Autodesk Inventor part; units mm, degrees
ref_plane "YZ Plane" through (0, 0, 0) normal (1, 0, 0) x (0, 1, 0)
ref_plane "XZ Plane" through (0, 0, 0) normal (0, 1, 0) x (-1, 0, 0)
ref_plane "XY Plane" through (0, 0, 0) normal (0, 0, 1) x (1, 0, 0)
sketch "Sketch1" plane through (0, 0, 0) normal (0, 0, 1) x (1, 0, 0)
  line L0 (0, 0) -> (80, 0)
  line L1 (80, 0) -> (80, 50)
  line L2 (80, 50) -> (0, 50)
  line L3 (0, 50) -> (0, 0)
  line L4 (15, 50) -> (65, 50)
  line L5 (65, 50) -> (65, 45)
  line L6 (65, 45) -> (15, 45)
  line L7 (15, 45) -> (15, 50)
  line L8 (5, 40) -> (75, 40)
  line L9 (75, 40) -> (75, 5)
  line L10 (75, 5) -> (5, 5)
  line L11 (5, 5) -> (5, 40)
  line L12 (-10, 0) -> (90, 0)
  line L13 (90, 0) -> (90, 5)
  line L14 (90, 5) -> (-10, 5)
  line L15 (-10, 5) -> (-10, 0)
  line L16 (0, 50) -> (5, 50)
  line L17 (5, 50) -> (5, 45)
  line L18 (5, 45) -> (0, 45)
  line L19 (0, 45) -> (0, 50)
  line L20 (80, 50) -> (75, 50)
  line L21 (75, 50) -> (75, 45)
  line L22 (75, 45) -> (80, 45)
  line L23 (80, 45) -> (80, 50)
  line L24 (37.5, 40) -> (42.5, 40)
  line L25 (42.5, 40) -> (42.5, 5)
  line L26 (42.5, 5) -> (37.5, 5)
  line L27 (37.5, 5) -> (37.5, 40)
  point P0 (40, 50)
  point P1 (40, 5)
  point P2 (40, 0)
  point P3 (40, 40)
  dimension "d0" = 80
  dimension "d1" = 50
  dimension "d2" = 50
  dimension "d3" = 70
  dimension "d4" = 100
  dimension "d5" = 5
  dimension "d6" = 5
  dimension "d7" = 5
  dimension "d10" = 5
  dimension "d11" = 5
  dimension "d12" = 5
extrude "Extrusion1" add sketch "Sketch1" along normal blind 10 contours L3 L14 L10 L1 L0 | L12 L15 L14 L3 | L1 L14 L13 L12 | L3 L18 L17 L2 L7 L6 L5 L21 L22 L1 L14 L9 L8 L11 | L27 L8 L25 L10
sketch "Sketch2" plane through (5, 50, 0) normal (0, 1, 0) x (1, 0, 0)
  line L0 (10, 0) -> (0, 0)
  circle A0 centre (5, -5) radius 1.7
  circle A1 centre (-10, -5) radius 1.7
  circle A2 centre (65, -5) radius 1.7
  circle A3 centre (80, -5) radius 1.7
  line L1 (70, -10) -> (70, 0)
  line L2 (70, 0) -> (60, 0)
  line L3 (85, 0) -> (75, 0)
  line L4 (-5, 0) -> (-15, 0)
  point P0 (70, -5)
  point P1 (5, 0)
  point P2 (65, 0)
  point P3 (80, 0)
  point P4 (-10, 0)
  dimension "d13" = 3.4
extrude "Extrusion2" cut sketch "Sketch2" against normal through all
sketch "Sketch3" plane through (5, 40, 10) normal (0, -1, 0) x (1, 0, 0)
  circle A0 centre (5, -5) radius 1.7
  circle A1 centre (5, -5) radius 3
  circle A2 centre (65, -5) radius 1.7
  circle A3 centre (65, -5) radius 3
  point P0 (-5, -10)
  dimension "d17" = 6
  dimension "d18" = 6
extrude "Extrusion3" cut sketch "Sketch3" against normal blind 3
properties part number "brush holder stand v5"
The listing builds one solid part. Answer for the finished solid, in the listing's coordinates (mm). A direction names the side the tool comes from. Give positions to 0.01 mm unless a question says otherwise; leave off trailing zeros. Write each loop counter-clockwise with the first axis right and the second up, starting at its lowest first coordinate (ties: lowest second). Pieces come first, ordered by that corner, then holes. Notation, with made-up numbers: (22, 10.25) -> (74, 10.25) arc R26 cw to (74, 33.25) -> close; hole circle Ø10 at (-33.5, 80). An arc over 180 degrees is marked (long way). Write item = value, one per line. Start each with the question number.
1) Straight lines are drawn through the part: line 1 along X through (y, z) = (17.5, 3.25); line 2 along X through (y, z) = (3.2, 5); line 3 along X through (y, z) = (45.5, 2.75). For each, find the intervals that lie inside material, in ascending order.
2) The part is cut by section B-B, the plane y = 3. Determine the outline of the cut face in (x, z).
3) Which of the six approach directions +Z, -Z, +X, -X, +Y, -Y give full straight-line access (tool end or side, diameter ignored) to faces 4 (the face through (37.5, 22, 5)), 5 (the face through (70, 43, 3)), 6 (the face through (77, 45, 5))?
4) Each of these flat-tipped pins is pushed along its axis until it touches: pin 1 (2.5 mm diameter, centred on y = 46.5, z = 3, fed in from -X); pin 2 (3 mm diameter, centred on x = 33, z = 7, fed in from +Y); pin 3 (3 mm diameter, centred on y = 15.5, z = 2.5, fed in from +X); pin 4 (2.5 mm diameter, centred on x = 10, z = 5, fed in from +Y). Where does it stop, or does it pass through?
5) The part is cut by section A-A, the plane x = 24. Determine the outline of the cut face in (y, z).
6) The part is cut by section C-C, the plane x = 10. Determine the outline of the cut face in (y, z).
7) The part is cut by section D-D, the plane y = 11.5. Determine the outline of the cut face in (x, z).
8) Determine the mould class of faces 1 (the face through (39, 0, 5)), 2 (the face through (-10, 3, 5)), 3 (the face through (68.3, 2.53, 4.93)) for opening direction X: +X half, -X half, draft (parallel to the pull), parting line (faces both ways), or undercut.
Solutions:
q1.line_1 = 0 to 5, 37.5 to 42.5, 75 to 80
q1.line_2 = -10 to -6.7, -3.3 to 8.3, 11.7 to 68.3, 71.7 to 83.3, 86.7 to 90
q1.line_3 = 5 to 15, 65 to 75
q2.outline = (-10, 0) -> (90, 0) -> (90, 10) -> (-10, 10) -> close; hole circle Ø3.4 at (-5, 5); hole circle Ø3.4 at (10, 5); hole circle Ø3.4 at (70, 5); hole circle Ø3.4 at (85, 5)
q3.face_4 = +Z, -Z
q3.face_5 = none
q3.face_6 = +Z, -Z, +X, +Y
q4.pin_1 = 5
q4.pin_2 = 45
q4.pin_3 = 80
q4.pin_4 = through
q5.outline = (0, 0) -> (5, 0) -> (5, 10) -> (0, 10) -> close; (40, 0) -> (45, 0) -> (45, 10) -> (40, 10) -> close
q6.outline = (0, 0) -> (5, 0) -> (5, 3.3) -> (0, 3.3) -> close; (0, 6.7) -> (5, 6.7) -> (5, 10) -> (0, 10) -> close; (40, 0) -> (50, 0) -> (50, 3.3) -> (43, 3.3) -> (43, 2) -> (40, 2) -> close; (40, 8) -> (43, 8) -> (43, 6.7) -> (50, 6.7) -> (50, 10) -> (40, 10) -> close
q7.outline = (0, 0) -> (5, 0) -> (5, 10) -> (0, 10) -> close; (37.5, 0) -> (42.5, 0) -> (42.5, 10) -> (37.5, 10) -> close; (75, 0) -> (80, 0) -> (80, 10) -> (75, 10) -> close
q8.face_1 = draft
q8.face_2 = -X half
q8.face_3 = undercut
